from build123d import *

# Parameters (mm, degrees)
SKETCH2_OUTSIDE_W  = 13.478
SKETCH2_OUTSIDE_H  = 13.478
CUT_EXTRUDE2_DEPTH = 10
CHAMFER1_SIZE      = 0.5
SKETCH3_R          = 0.2
CUT_EXTRUDE3_DEPTH = 15.102688869


with BuildPart() as part:
    # Sketch1 → Revolve1 (revolve)
    with BuildSketch(Plane(origin=(0, 0, 0), x_dir=(1, 0, 0), z_dir=(0, 1, 0)), mode=Mode.PRIVATE) as revolve1_sk:
        Polygon((1, 8.7), (3, 8.7), (3, 3.5), (4, 3.5), (4, 0), (0.85, -4.5), (0, -4.5), (0, -3.673205081), (1, -1.941154273), align=None)
    revolve(revolve1_sk.sketch.rotate(Axis((0, 0, 0), (0, 0, 1)), 180), axis=Axis((0, 0, 0), (0, 0, 1)))

    # Sketch2 outside → Cut-Extrude2 (cut)
    with BuildSketch(Plane(origin=(0, 0, -3.5), x_dir=(-1, 0, 0), z_dir=(0, 0, -1))):
        Rectangle(SKETCH2_OUTSIDE_W, SKETCH2_OUTSIDE_H)
        Polygon((3.25, 1.876388375), (0, 3.75277675), (-3.25, 1.876388375), (-3.25, -1.876388375), (0, -3.75277675), (3.25, -1.876388375), align=None, mode=Mode.SUBTRACT)
    extrude(amount=-CUT_EXTRUDE2_DEPTH, mode=Mode.SUBTRACT)

    # Chamfer1
    chamfer1_edges = [part.edges().sort_by_distance(p)[0] for p in [
        (3, 0, -8.7),
    ]]
    chamfer(chamfer1_edges, length=CHAMFER1_SIZE)

    # Sketch3 → Cut-Extrude3 (cut, through all)
    with BuildSketch(Plane.XY.offset(4.5)):
        Circle(SKETCH3_R)
    extrude(amount=-CUT_EXTRUDE3_DEPTH, mode=Mode.SUBTRACT)


solid = part.part
CAD build for the part. Positions are in the model's coordinates, mm. A direction names the side the tool comes from. Round coordinates to 2 decimals unless told otherwise and drop trailing zeros. Write each loop counter-clockwise with the first axis right and the second up, starting at its lowest first coordinate (ties: lowest second). Pieces come first, ordered by that corner, then holes.
(1) Drop flat-ended pins along their axis: P1, Ø1.5, axis at x = 0, z = 2, coming from the -Y side (3 decimals); P2, Ø2, axis at x = -1.5, z = -6.5, coming from the +Y side. Give the stop position or say it passes through.
(2) Slice it at C-C, the plane z = -4.5. Write the cut outline in (x, y), and give its area (3 significant figures).
(3) 3-axis set-ups, long thin cutter, end or side, ignore diameter. For faces 1 (the face through (-1, 3, -3.5)), 2 (the face through (3.25, 0, -1)): which of +Z, -Z, +X, -X, +Y, -Y reach the whole face in a straight line?
(4) Slice it at D-D, the plane z = 2.25. Write the cut outline in (x, y) (3 decimals).
(5) Probe line 1 along Y through (x, z) = (0, -6); line 2 along X through (y, z) = (0.75, -3); line 3 along Y through (x, z) = (-0.75, -0.75). List the from-to ranges inside material, lowest first.
(6) Slice it at A-A, the plane y = 0. Write the cut outline in (x, z).
(7) Mould opens along Y. For faces 3 (the face through (-1.6, -2.83, -1.25)), 4 (the face through (1, 1, -8.7)), 5 (the face through (0.34, 0.26, 2.93)) say: pulls with the +Y half, pulls with the -Y half, needs draft (parallel to the pull), parting line crosses it, or undercut.
(8) Slice it at B-B, the plane z = 0. Write the cut outline in (x, y), and give its area (3 significant figures).
From the geometry:
1. P1: stops at y = -3.125
1. P2: stops at y = 2.96
2. outline: circle Ø6 at (0, 0); hole circle Ø2 at (0, 0)
2. area: 25.1 mm2
3. face 1: -Z
3. face 2: +Z, -Z, +X, +Y, -Y
4. outline: circle Ø4.85 at (0, 0); hole circle Ø1.643 at (0, 0)
5. line 1: y = -3 to -1, 1 to 3
5. line 2: x = -3.25 to -0.66, 0.66 to 3.25
5. line 3: y = -3.32 to -0.66, 0.66 to 3.32
6. outline: (-3.25, -3.5) - (-3, -3.5) - (-3, -8.2) - (-2.5, -8.7) - (-1, -8.7) - (-1, 1.94) - (-0.2, 3.33) - (-0.2, 4.5) - (-0.85, 4.5) - (-3.25, 1.07) - close; (0.2, 3.33) - (1, 1.94) - (1, -8.7) - (2.5, -8.7) - (3, -8.2) - (3, -3.5) - (3.25, -3.5) - (3.25, 1.07) - (0.85, 4.5) - (0.2, 4.5) - close
7. face 3: pulls with the -Y half
7. face 4: needs draft
7. face 5: undercut
8. outline: (-3.25, -1.88) - (0, -3.75) - (3.25, -1.88) - (3.25, 1.88) - (0, 3.75) - (-3.25, 1.88) - close; hole circle Ø2 at (0, 0)
8. area: 33.4 mm2
